```python
from build123d import *

# Parameters (mm, degrees)
F0_W     = 152.4
F0_H     = 342.9
F1_DEPTH = 4.7625
F2_W     = 25.4
F2_H     = 4.7625
F3_DEPTH = 9.525
F4_W     = 152.4
F4_H     = 4.7625
F5_DEPTH = 9.525
F6_W     = 12.7
F6_H     = 241.3
F7_DEPTH = 4.7625


with BuildPart() as f1:
    # F0 (on Front) → F1 (new body)
    with BuildSketch(Plane.XZ):
        Rectangle(F0_W, F0_H)
    extrude(amount=F1_DEPTH)

    # F2 (on face) → F3 (join)
    with BuildSketch(Plane.XZ.offset(4.7625)):
        with Locations((-50.8, 169.06875)):
            Rectangle(F2_W, F2_H)
        with Locations((50.8, 169.06875)):
            Rectangle(F2_W, F2_H)
    extrude(amount=-F3_DEPTH)

    # F4 (on face) → F5 (join)
    with BuildSketch(Plane.XZ.offset(4.7625)):
        with Locations((0, -169.06875)):
            Rectangle(F4_W, F4_H)
    extrude(amount=-F5_DEPTH)

    # F6 (on Front) → F7 (join)
    with BuildSketch(Plane.XZ):
        with Locations((-69.85, 292.1)):
            Rectangle(F6_W, F6_H)
        with Locations((69.85, 292.1)):
            Rectangle(F6_W, F6_H)
    extrude(amount=F7_DEPTH)


solid = f1.part
```
Source: CAD feature listing. Evaluate the final solid. Frame: model axes, mm. Coordinates: 2 decimals unless noted, no trailing zeros. Write each loop counter-clockwise with the first axis right and the second up, starting at its lowest first coordinate (ties: lowest second). Pieces come first, ordered by that corner, then holes. Notation, with made-up numbers: M 10,29.25 L 42,29.25 A31 cw 42,63.25 Z; hole C 6.5,51.25 d7. An arc over 180 degrees is marked long. Answer as a JSON object with one key per item and string values.
1. Cut plane B-B on y = 3.25. Output: boundary loops of the cut face in (x, z), plus the area to 3 significant figures.
Evaluation:
{"outline": "M -76.2,-171.45 L 76.2,-171.45 L 76.2,-166.69 L -76.2,-166.69 Z; M -63.5,166.69 L -38.1,166.69 L -38.1,171.45 L -63.5,171.45 Z; M 38.1,166.69 L 63.5,166.69 L 63.5,171.45 L 38.1,171.45 Z", "area": "968 mm^2"}
2. Draft query along X for faces 1 (the flat face through (-1, -4.762, 60)), 2 (the flat face through (76.2, -2, 117)), 3 (the flat face through (-76.2, -2, 117)), 4 (the flat face through (-1, -1, 171.45)). Return one class per face: released by +X, released by -X, zero draft, split by the parting line, or undercut.
Evaluation:
{"face 1": "zero draft", "face 2": "released by +X", "face 3": "released by -X", "face 4": "undercut"}
3. Cut plane D-D on z = 121. Output: boundary loops of the cut face in (x, y), plus the area to 3 significant figures.
Evaluation:
{"outline": "M -76.2,-4.76 L 76.2,-4.76 L 76.2,0 L -76.2,0 Z", "area": "726 mm^2"}
4. Contact query for flat-ended pins moving along their axis: P1, Ø4, axis at x = -12, y = 2.5, coming from the +Z side; P2, Ø6, axis at x = 15.5, z = 121.5, coming from the +Y side; P3, Ø1.4, axis at y = 1.5, z = 169.5, coming from the +X side. Output: stop coordinate, or through.
Evaluation:
{"P1": "z = -166.69", "P2": "y = 0", "P3": "x = 63.5"}
5. Ray query, L1, parallel to X at y = -3.25, z = 189; L2, parallel to Z at x = 62.5, y = 3.5; L3, parallel to Z at x = -15, y = 3.5. Return the intervals inside material, ascending.
Evaluation:
{"L1": "-76.2 to -63.5, 63.5 to 76.2", "L2": "-171.45 to -166.69, 166.69 to 171.45", "L3": "-171.45 to -166.69"}
6. Cut plane C-C on x = -47. Output: boundary loops of the cut face in (y, z).
Evaluation:
{"outline": "M -4.76,-171.45 L 4.76,-171.45 L 4.76,-166.69 L 0,-166.69 L 0,166.69 L 4.76,166.69 L 4.76,171.45 L -4.76,171.45 Z"}
7. Cut plane A-A on z = 311. Output: boundary loops of the cut face in (x, y), plus the area to 3 significant figures.
Evaluation:
{"outline": "M -76.2,-4.76 L -63.5,-4.76 L -63.5,0 L -76.2,0 Z; M 63.5,-4.76 L 76.2,-4.76 L 76.2,0 L 63.5,0 Z", "area": "121 mm^2"}
